Here's how the part is built. I have some questions about the finished solid (model axes, mm). Give positions to 0.01 mm unless a question says otherwise; leave off trailing zeros. Write each loop counter-clockwise with the first axis right and the second up, starting at its lowest first coordinate (ties: lowest second). Pieces come first, ordered by that corner, then holes. Notation, with made-up numbers: M -5.5,-8 L 35.5,-8 A19 cw 35.5,27 Z; hole C -11,16.5 d2. An arc over 180 degrees is marked long. Answer as CSV lines item,"result". Start each with the question number.
Q1. For pin 1 (2 mm diameter, centred on x = 2.5, y = -85.5, fed in from +Z); pin 2 (1 mm diameter, centred on x = 2, y = 15.5, fed in from -Z), each with a flat end and sliding along its axis, tell me the tip position at first contact or that it passes through.
Q2. Suppose I cut it at B-B (y = -114). Write out the boundary of the cut face in (x, z), then the cut area to 3 significant figures.
Q3. If I drill on line 1 along X through (y, z) = (112.5, 0.95); line 2 along X through (y, z) = (22, 0.5); line 3 along Z through (x, y) = (2.3, 119.5), over which ranges is the centre line in solid material (lowest first)?
Q4. Suppose I cut it at A-A (y = 27.5). Write out the boundary of the cut face in (x, z), then the cut area to 3 significant figures.
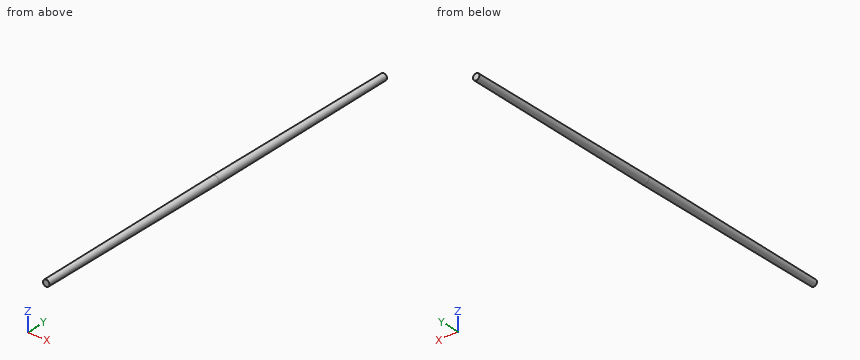
```python
from build123d import *

# Parameters (mm, degrees)
ECHELLE1_SCALE = 0.6


with BuildPart() as part:
    # Esquisse1 → Révolution1 (revolve)
    with BuildSketch(Plane.XY, mode=Mode.PRIVATE) as r_volution1_sk:
        Polygon((0, 0), (5, 0), (4, 250), (0, 250), align=None)
    r_volution1 = revolve(r_volution1_sk.sketch.rotate(Axis((0, 250, 0), (0, -1, 0)), 180), axis=Axis((0, 250, 0), (0, -1, 0)))

    # Symétrie1: Révolution1 across plane
    add(r_volution1.mirror(Plane.ZX))


with BuildPart() as part_1:
    # Echelle1: scaled about (0, 0, 0)
    add(part.part.scale(ECHELLE1_SCALE))


solid = part_1.part
```
Resolved:
1,pin 1,"z = 2.19"
1,pin 2,"z = -2.53"
2,outline,"C 0,0 d5.09"
2,area,"20.3 mm^2"
3,line 1,"-2.37 to 2.37"
3,line 2,"-2.87 to 2.87"
3,line 3,"-1.03 to 1.03"
4,outline,"C 0,0 d5.78"
4,area,"26.2 mm^2"
